from build123d import *

# Parameters (mm, degrees)
F0_R     = 4
F1_DEPTH = 135


# Not quite as in the source:
# - a feature names something its author has since deleted; it is built from what else it names


with BuildPart() as f1:
    # F0 (on Top) → F1 (new body)
    with BuildSketch(Plane.XY):
        Circle(F0_R)
    extrude(amount=F1_DEPTH)


with BuildPart() as f3:
    # F2 (on Front) → F3 (revolve)
    with BuildSketch(Plane.XZ):
        with BuildLine():
            ThreePointArc((-5.4025318968, 144.3044847424), (-8.7187941889, 142.570608457), (-10.4812420468, 139.2694419797))
            Line((-10.4812420468, 139.2694419797), (-10.4812420468, 137.5795906956))
            Line((-10.4812420468, 137.5795906956), (-7.6773734327, 137.5795906956))
            Line((-7.6773734327, 137.5795906956), (-7.6773734327, 136.4770686801))
            Line((-7.6773734327, 136.4770686801), (-10.4469684447, 136.4770686801))
            Line((-10.4469684447, 136.4770686801), (-10.4469684447, 135.2973152099))
            Line((-10.4469684447, 135.2973152099), (-7.5175449747, 135.319129246))
            Line((-7.5175449747, 135.319129246), (-7.5175449747, 134.2156535561))
            Line((-7.5175449747, 134.2156535561), (-10.4518206354, 134.2156535561))
            Line((-10.4518206354, 134.2156535561), (-10.4518206354, 133.2342779811))
            Line((-10.4518206354, 133.2342779811), (-7.5175449747, 133.2342779811))
            Line((-7.5175449747, 133.2342779811), (-7.4386694032, 131.9274908478))
            Line((-7.4386694032, 131.9274908478), (-10.4812420468, 131.9274908478))
            Line((-10.4812420468, 131.9274908478), (-10.4812420468, 130.9773630078))
            Line((-10.4812420468, 130.9773630078), (-7.5752432022, 130.9773630078))
            Line((-7.5752432022, 130.9773630078), (-7.5752432022, 129.9533254082))
            Line((-7.5752432022, 129.9533254082), (-10.4812420468, 129.9533254082))
            Line((-10.4812420468, 129.9533254082), (-10.4812420468, 128.8439488585))
            Line((-10.4812420468, 128.8439488585), (-7.4899065803, 128.8439488585))
            Line((-7.4899065803, 128.8439488585), (-7.4899065803, 127.4785554583))
            Line((-7.4899065803, 127.4785554583), (-10.4812420468, 127.4785554583))
            Line((-10.4812420468, 127.4785554583), (-10.4812420468, 126.3265168841))
            Line((-10.4812420468, 126.3265168841), (-7.4899065803, 126.3265168841))
            Line((-7.4899065803, 126.3265168841), (-7.4899065803, 125.3024643834))
            Line((-7.4899065803, 125.3024643834), (-10.4812420468, 125.3024643834))
            Line((-10.4812420468, 125.3024643834), (-10.4812420468, 124.2357573087))
            Line((-10.4812420468, 124.2357573087), (-7.8191701323, 124.2357573087))
            Line((-7.8191701323, 124.2357573087), (-7.8191701323, 123.4466135502))
            Line((-7.8191701323, 123.4466135502), (-10.4812420468, 123.4466135502))
            Line((-10.4812420468, 123.4466135502), (-10.4812420468, 122.4818459327))
            Line((-10.4812420468, 122.4818459327), (-7.861838676, 122.4818459327))
            Line((-7.861838676, 122.4818459327), (-7.861838676, 121.4195713401))
            Line((-7.861838676, 121.4195713401), (-10.7123531493, 121.4195713401))
            ThreePointArc((-10.7123531493, 121.4195713401), (-8.6638063846, 118.8171942191), (-5.8128938955, 117.1316057444))
            Line((-5.8128938955, 117.1316057444), (-5.5729771993, 117.1316057444))
            Line((-5.5729771993, 117.1316057444), (-5.5729771993, 107.9735688748))
            Line((-5.5729771993, 107.9735688748), (-9.4849373709, 107.9735688748))
            Line((-9.4849373709, 107.9735688748), (-9.4849373709, 103.0133224906))
            Line((-9.4849373709, 103.0133224906), (0, 103.0133224906))
            Line((0, 103.0133224906), (0, 144.3145008144))
            Line((0, 144.3145008144), (-5.4025318968, 144.3044847424))
        make_face()
    revolve(axis=Axis((0, 0, 123.6639116525), (0, 0, 1)))

    # F4: cut F1
    add(f1.part, mode=Mode.SUBTRACT)


solid = f3.part
Design review of the part built by this model. Coordinates are the model's own, in mm. A direction names the side the tool comes from. Coordinates: 2 decimals unless noted, no trailing zeros. Order: outer loops, then holes, each group sorted by start corner. A loop starts at its lowest first (then second) coordinate and runs counter-clockwise, first axis right, second up. Notation, with made-up numbers: (1.25, 42) -> (59.25, 42) arc R32 ccw to (59.25, 68) -> close; hole circle Ø9 at (59.5, 26.5). An arc over 180 degrees is marked (long way). Use one line per item in the form item = value. Start each with the question number.
(1) For faces 1 (the cylindrical face through (7.53, 5.77, 105.46)), 2 (the flat face through (8, 1, 124.236)), list the 3-axis set-ups (+Z, -Z, +X, -X, +Y, -Y) from which the entire face can be reached by the end or side of a thin tool; tool diameter is ignored.
(2) Add section B-B on z = 131.5. State the section outline as (x, y) points, plus the area to 3 significant figures.
(3) For probe 1 along Y at (x, z) = (0, 121); probe 2 along X at (y, z) = (0, 128.5); probe 3 along Y at (x, z) = (0, 114), list the stretches that pass through material, from the lowest coordinate up.
(4) Insertion check: pin 1 (1 mm diameter, centred on y = 3, z = 127.5, fed in from -X); pin 2 (6 mm diameter, centred on x = -0.5, z = 118, fed in from -Y); pin 3 (1 mm diameter, centred on x = 4.5, z = 131.5, fed in from -Y). Each pin has a flat end and moves straight along its axis. Give the tip position at first contact, or say it passes through.
(5) The part is to be moulded in two halves that separate along Z. For faces 3 (the flat face through (5, 7, 125.302)), 4 (the cylindrical face through (1.364, -10.392, 126.894)), 5 (the flat face through (-2, 4, 103.013)), say which applies: +Z half, -Z half, draft (parallel to the pull), parting line (faces both ways), or undercut.
(6) Add section A-A on z = 122. State the section outline as (x, y) points, plus the area to 3 significant figures.
Answer block:
q1.face_1 = -Z
q1.face_2 = none
q2.outline = circle Ø20.96 at (0, 0); hole circle Ø8 at (0, 0)
q2.area = 295 mm²
q3.probe_1 = -10.48 to -4, 4 to 10.48
q3.probe_2 = -7.49 to -4, 4 to 7.49
q3.probe_3 = -5.57 to -4, 4 to 5.57
q4.pin_1 = -10.18
q4.pin_2 = -10.47
q4.pin_3 = -9.69
q5.face_3 = undercut
q5.face_4 = draft
q5.face_5 = -Z half
q6.outline = circle Ø15.72 at (0, 0); hole circle Ø8 at (0, 0)
q6.area = 144 mm²
